Source: CAD feature listing. Evaluate the final solid. Frame: model axes, mm. Face numbers are marked on the shaded views. A direction names the side the tool comes from. Give positions to 0.01 mm unless a question says otherwise; leave off trailing zeros. Loops run counter-clockwise (first coordinate to the right, second up) from the corner with the lowest first, then second, coordinate; pieces in that order, holes last. Notation, with made-up numbers: M 89,9.25 L 117,9.25 A19 ccw 117,46.25 Z; hole C 23,-14.75 d4. An arc over 180 degrees is marked long. Answer in a Markdown table with one row per item.
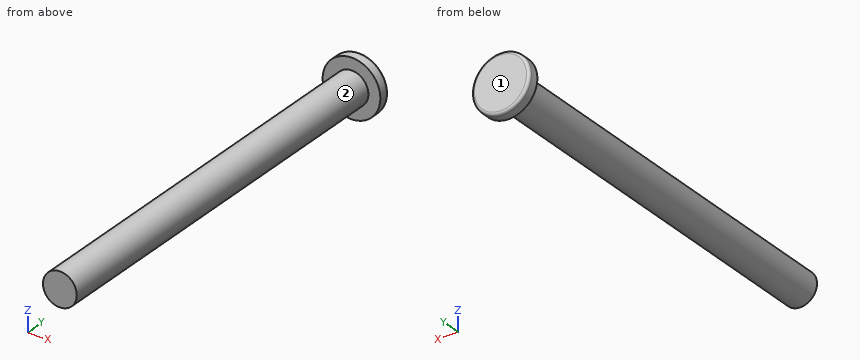
```python
from build123d import *

# Parameters (mm, degrees)
F0_R     = 20.5
F0_R_2   = 12
F1_DEPTH = 8
F2_DEPTH = 300
F3_R     = 2


with BuildPart() as f1:
    # F0 (on Front) → F1 (new body)
    with BuildSketch(Plane.XZ):
        Circle(F0_R)
        Circle(F0_R_2, mode=Mode.SUBTRACT)
        Circle(F0_R_2)
    extrude(amount=F1_DEPTH)

    # F0 (on Front) → F2 (join)
    with BuildSketch(Plane.XZ):
        Circle(F0_R_2)
    extrude(amount=F2_DEPTH)

    # F3
    f3_edges = [f1.edges().sort_by_distance(p)[0] for p in [
        (-20.5, 0, 0),
    ]]
    fillet(f3_edges, radius=F3_R)


solid = f1.part
```
Q1. Contact query for flat-ended pins moving along their axis: pin 1 Ø8 at (x, z) = (-0.5, 3) entering from +Y; pin 2 Ø1.5 at (x, y) = (-14.5, -261.5) entering from +Z; pin 3 Ø4 at (y, z) = (-176.5, 10) entering from +X; pin 4 Ø2 at (x, z) = (-7.5, -15.5) entering from -Y. Output: stop coordinate, or through.
Values follow:
| item | result |
|---|---|
| pin 1 | y = 0 |
| pin 2 | through |
| pin 3 | x = 8.94 |
| pin 4 | y = -8 |
Q2. Section query B-B (z = 0). Output: boundary loops of the cut face in (x, y).
Values follow:
| item | result |
|---|---|
| outline | M -20.5,-8 L -12,-8 L -12,-300 L 12,-300 L 12,-8 L 20.5,-8 L 20.5,-2 A2 ccw 18.5,0 L -18.5,0 A2 ccw -20.5,-2 Z |
Q3. Section query C-C (y = -209.5). Output: boundary loops of the cut face in (x, z), plus the area to 3 significant figures.
Values follow:
| item | result |
|---|---|
| outline | C 0,0 d24 |
| area | 452 mm^2 |
Q4. Section query A-A (x = 0). Output: boundary loops of the cut face in (y, z), plus the area to 3 significant figures.
Values follow:
| item | result |
|---|---|
| outline | M -300,-12 L -8,-12 L -8,-20.5 L -2,-20.5 A2 ccw 0,-18.5 L 0,18.5 A2 ccw -2,20.5 L -8,20.5 L -8,12 L -300,12 Z |
| area | 7,330 mm^2 |
Q5. Ray query, probe 1 along Y at (x, z) = (-15.5, 0.5); probe 2 along X at (y, z) = (-232.5, -1); probe 3 along X at (y, z) = (-13, -11). Return the intervals inside material, ascending. Write a range as from..to.
Values follow:
| item | result |
|---|---|
| probe 1 | -8..0 |
| probe 2 | -11.96..11.96 |
| probe 3 | -4.8..4.8 |
Q6. Reachability of the marked faces 1 and 2 from +Z, -Z, +X, -X, +Y, -Y: full face, straight path, thin tool, end or side. Return the list, or none.
Values follow:
| item | result |
|---|---|
| face 1 | +Z, -Z, +X, -X, +Y |
| face 2 | -Y |
